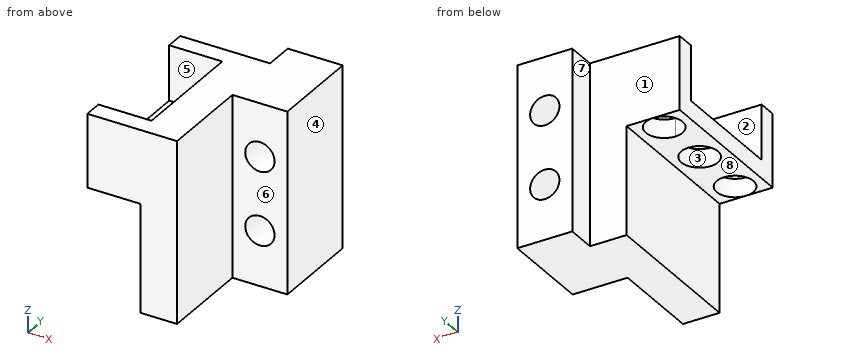
from build123d import *

# Parameters (mm, degrees)
SKETCH077_W            = 20
SKETCH077_H            = 19.8
PAD046_DEPTH           = 6
SKETCH078_R            = 1.6
POCKET032_DEPTH        = 40
SKETCH079_W            = 16.8
SKETCH079_H            = 19.8
PAD047_DEPTH           = 4
PAD048_DEPTH           = 5.8
SKETCH081_R            = 2
POCKET033_DEPTH        = 5
LINEARPATTERN002_COUNT = 3
LINEARPATTERN002_PITCH = 6.4
SKETCH082_W            = 19.8
SKETCH082_H            = 6
POCKET034_DEPTH        = 10


with BuildPart() as part:
    # Sketch077 → Pad046 (new body)
    with BuildSketch(Plane.YZ):
        with Locations((-6, 0.1)):
            Rectangle(SKETCH077_W, SKETCH077_H)
    extrude(amount=PAD046_DEPTH)

    # Sketch078 (on Face4 of Pad046) → Pocket032 (cut)
    with BuildSketch(Plane(origin=(0, -16, 0), x_dir=(0, 0, -1), z_dir=(0, -1, 0))):
        with Locations((3.8, 3)):
            Circle(SKETCH078_R)
        with Locations((-4.2, 3)):
            Circle(SKETCH078_R)
    extrude(amount=-POCKET032_DEPTH, mode=Mode.SUBTRACT)

    # Sketch079 (on Face4 of Pocket032) → Pad047 (join)
    with BuildSketch(Plane(origin=(0, 0, 0), x_dir=(0, 1, 0), z_dir=(-1, 0, 0))):
        with Locations((-7.6, -0.1)):
            Rectangle(SKETCH079_W, SKETCH079_H)
    extrude(amount=PAD047_DEPTH)

    # Sketch080 (on Face7 of Pad047) → Pad048 (join)
    with BuildSketch(Plane(origin=(-4, 0, 0), x_dir=(0, 1, 0), z_dir=(-1, 0, 0))):
        Polygon((-16, -10), (-16, -2), (0.8, -2), (0.8, -10), (-1.2, -10), (-1.2, -4), (-14, -4), (-14, -10), align=None)
    extrude(amount=PAD048_DEPTH)

    # Sketch081 (on Face13 of Pad048) → Pocket033 (cut)
    with BuildSketch(Plane(origin=(0, 0, 4), x_dir=(0, -1, 0), z_dir=(0, 0, 1))):
        with Locations((1.2, -6.9)):
            Circle(SKETCH081_R)
    pocket033 = extrude(amount=-POCKET033_DEPTH, mode=Mode.SUBTRACT)

    # LinearPattern002: Pocket033 ×3
    with Locations(*[(0, -i * LINEARPATTERN002_PITCH, 0) for i in range(1, LINEARPATTERN002_COUNT)]):
        add(pocket033, mode=Mode.SUBTRACT)

    # Sketch082 (on Face8 of LinearPattern002) → Pocket034 (cut)
    with BuildSketch(Plane(origin=(0, -16, 0), x_dir=(0, 0, -1), z_dir=(0, -1, 0))):
        with Locations((-0.1, 3)):
            Rectangle(SKETCH082_W, SKETCH082_H)
    extrude(amount=-POCKET034_DEPTH, mode=Mode.SUBTRACT)


with BuildPart() as part_1:
    # Body012 placement: moved
    add(part.part.moved(Location((26, -13, -16.3))))


solid = part_1.part
Read the model definition and answer for the solid it produces. Units are mm, in the model's axes. Face numbers are marked on the shaded views. A direction names the side the tool comes from. Round coordinates to 2 decimals unless told otherwise and drop trailing zeros. Write each loop counter-clockwise with the first axis right and the second up, starting at its lowest first coordinate (ties: lowest second). Pieces come first, ordered by that corner, then holes.
1. Determine the mould class of the marked faces 1, 2, 3 and 4 for opening direction Y: pulls with the +Y half, pulls with the -Y half, needs draft (parallel to the pull), parting line crosses it, or undercut.
2. Which of the six approach directions +Z, -Z, +X, -X, +Y, -Y give full straight-line access (tool end or side, diameter ignored) to the marked faces 5, 6, 7 and 8?
3. Given pin 1 Ø1.7 at (x, y) = (18.5, -17.5) entering from -Z; pin 2 Ø6 at (y, z) = (-17.5, -18) entering from -X; pin 3 Ø1.5 at (y, z) = (-22, -10) entering from +X; pin 4 Ø2.5 at (x, z) = (29, -20.1) entering from +Y, each flat-ended and moving along its own axis, determine where each tip first touches the part or whether it passes through.
4. The part is cut by section D-D, the plane y = -15. Determine the outline of the cut face in (x, z), then the cut area to 3 significant figures.
5. The part is cut by section B-B, the plane x = 29. Determine the outline of the cut face in (y, z), then the cut area to 3 significant figures.
6. Straight lines are drawn through the part: L1, parallel to X at y = -12.5, z = -12.1; L2, parallel to X at y = -27, z = -13.25; L3, parallel to Z at x = 30, y = -14.25. For each, find the intervals that lie inside material, in ascending order.
7. The part is cut by section A-A, the plane z = -20.1. Determine the outline of the cut face in (x, y), then the cut area to 3 significant figures.
Values:
1. face 1: pulls with the +Y half
1. face 2: undercut
1. face 3: undercut
1. face 4: needs draft
2. face 5: +Z, -X
2. face 6: +Z, -Z, +X, -Y
2. face 7: +Z, -Z, -X, +Y
2. face 8: -Z, -X, +Y, -Y
3. pin 1: stops at z = -14.3
3. pin 2: stops at x = 22
3. pin 3: stops at x = 26
3. pin 4: passes through
4. outline: (16.2, -14.3) - (17.27, -14.3) - (17.27, -12.3) - (16.2, -12.3) - close; (20.93, -14.3) - (22, -14.3) - (22, -26.1) - (32, -26.1) - (32, -6.3) - (22, -6.3) - (22, -12.3) - (20.93, -12.3) - close; hole circle Ø3.2 at (29, -20.1); hole circle Ø3.2 at (29, -12.1)
4. area: 186 mm2
5. outline: (-19, -26.1) - (-9, -26.1) - (-9, -21.7) - (-19, -21.7) - close; (-19, -18.5) - (-9, -18.5) - (-9, -13.7) - (-19, -13.7) - close; (-19, -10.5) - (-9, -10.5) - (-9, -6.3) - (-19, -6.3) - close
5. area: 134 mm2
6. L1: x = 16.2 to 27.4, 30.6 to 32
6. L2: x = 16.2 to 17.1, 21.1 to 26
6. L3: z = -26.1 to -21.35, -18.85 to -13.35, -10.85 to -6.3
7. outline: (22, -29) - (26, -29) - (26, -19) - (27.4, -19) - (27.4, -9) - (26, -9) - (26, -12.2) - (22, -12.2) - close; (30.6, -19) - (32, -19) - (32, -9) - (30.6, -9) - close
7. area: 95.2 mm2
